from build123d import *

# Parameters (mm, degrees)
F0_W     = 19.05
F0_H     = 6.35
F1_DEPTH = 25.4
F2_W     = 19.05
F2_H     = 6.35
F3_DEPTH = 12.701
F4_W     = 19.05
F4_H     = 6.35
F5_DEPTH = 38.101
F6_R     = 3.175
F7_DEPTH = 12.7


with BuildPart() as f1:
    # F0 (on Front) → F1 (new body)
    with BuildSketch(Plane.XZ):
        Polygon((0, 12.7), (0, 0), (6.35, 0), (6.35, 6.35), (19.05, 6.35), (19.05, 12.7), align=None)
        Polygon((19.05, 25.4), (19.05, 12.7), (19.05, 6.35), (38.1, 6.35), (38.1, 12.7), (38.1, 25.4), align=None)
        with Locations((28.575, 28.575)):
            Rectangle(F0_W, F0_H)
    extrude(amount=F1_DEPTH)

    # F2 (on face) → F3 (cut, through all)
    with BuildSketch(Plane.XY.offset(12.7)):
        with Locations((9.525, -22.225)):
            Rectangle(F2_W, F2_H)
    extrude(amount=-F3_DEPTH, mode=Mode.SUBTRACT)

    # F4 (on face) → F5 (cut, through all)
    with BuildSketch(Plane.YZ.offset(38.1)):
        with Locations((-15.875, 28.575)):
            Rectangle(F4_W, F4_H)
    extrude(amount=-F5_DEPTH, mode=Mode.SUBTRACT)

    # F6 (on face) → F7 (cut, symmetric)
    with BuildSketch(Plane.XY.offset(12.7)):
        with Locations((29.162522, -17.198412)):
            Circle(F6_R)
        with Locations((12.71187, -10.361776)):
            Circle(F6_R)
    extrude(amount=F7_DEPTH, both=True, mode=Mode.SUBTRACT)


solid = f1.part
The model under review builds one solid part; all positions refer to its coordinate system, in mm. A direction names the side the tool comes from. Coordinates: 2 decimals unless noted, no trailing zeros. Write each loop counter-clockwise with the first axis right and the second up, starting at its lowest first coordinate (ties: lowest second). Pieces come first, ordered by that corner, then holes. Notation, with made-up numbers: (60.25, 85.25) - (107.25, 85.25) arc R20 cw to (107.25, 98.25) - close; hole circle Ø6 at (55, -38). An arc over 180 degrees is marked (long way). Answer as CSV lines item,"result".
(1) Mouldability with a two-part tool opening along X and no side actions: class faces 5 (the cylindrical face through (15.645, -11.578, 9.569)), 6 (the flat face through (0, -9, 6)), 7 (the flat face through (23, 0, 16)) as pulls with the +X half, pulls with the -X half, needs draft (parallel to the pull), parting line crosses it, or undercut.
Data:
face 5,"undercut"
face 6,"pulls with the -X half"
face 7,"needs draft"
(2) We need section A-A (y = -5.25). Give the boundary of the cut face in (x, z).
Data:
outline,"(0, 0) - (6.35, 0) - (6.35, 6.35) - (38.1, 6.35) - (38.1, 31.75) - (19.05, 31.75) - (19.05, 12.7) - (0, 12.7) - close"
(3) For line 1 along X through (y, z) = (-7.75, 18); line 2 along Z through (x, y) = (22, -14.5); line 3 along Y through (x, z) = (10, 6.5), list the stretches that pass through material, from the lowest coordinate up. Write a range as [from, to].
Data:
line 1,"x = [19.05, 38.1]"
line 2,"z = [6.35, 25.4]"
line 3,"y = [-19.05, -12.01], [-8.71, 0]"
(4) Clearance check with flat-ended pins moving along their axes: pin 1 Ø5 at (x, y) = (29.16, -17.2) entering from +Z; pin 2 Ø15 at (x, y) = (8.5, -11.5) entering from +Z; pin 3 Ø7.5 at (x, y) = (29.16, -17.2) entering from +Z; pin 4 Ø3 at (x, y) = (28, -3) entering from -Z. State where each tip first meets the part, or that it passes through.
Data:
pin 1,"passes through"
pin 2,"stops at z = 12.7"
pin 3,"stops at z = 25.4"
pin 4,"stops at z = 6.35"
(5) Tool access review of faces 1 (the flat face through (8, -9, 12.7)), 2 (the flat face through (7, -19.05, 8)), 3 (the flat face through (29, -6.35, 29)), 4 (the flat face through (22, -13, 6.35)): name each direction out of +Z, -Z, +X, -X, +Y, -Y from which nothing blocks a thin tool from reaching the whole face with its end or side.
Data:
face 1,"+Z, -X, +Y, -Y"
face 2,"+Z, -Z, -X, -Y"
face 3,"+Z, +X, -X, -Y"
face 4,"-Z, +X, +Y, -Y"
(6) We need section D-D (z = 10). Give the boundary of the cut face in (x, y) (3 decimals).
Data:
outline,"(0, -19.05) - (19.05, -19.05) - (19.05, -25.4) - (38.1, -25.4) - (38.1, 0) - (0, 0) - close; hole circle Ø6.35 at (12.712, -10.362); hole circle Ø6.35 at (29.163, -17.198)"
(7) We need section B-B (y = -15). Give the boundary of the cut face in (x, z).
Data:
outline,"(0, 0) - (6.35, 0) - (6.35, 6.35) - (26.87, 6.35) - (26.87, 25.4) - (19.05, 25.4) - (19.05, 12.7) - (0, 12.7) - close; (31.45, 6.35) - (38.1, 6.35) - (38.1, 25.4) - (31.45, 25.4) - close"
(8) We need section C-C (x = 10). Give the boundary of the cut face in (y, z), plus the area to 4 significant figures.
Data:
outline,"(-19.05, 6.35) - (-12.01, 6.35) - (-12.01, 12.7) - (-19.05, 12.7) - close; (-8.71, 6.35) - (0, 6.35) - (0, 12.7) - (-8.71, 12.7) - close"
area,"100.0 mm2"
